Geometry: final body of the model. Coordinates: model frame, mm. A direction names the side the tool comes from. Give positions to 0.01 mm unless a question says otherwise; leave off trailing zeros. Write each loop counter-clockwise with the first axis right and the second up, starting at its lowest first coordinate (ties: lowest second). Pieces come first, ordered by that corner, then holes.
```python
from build123d import *

# Parameters (mm, degrees)
SKETCH1_R                   = 8.89
BOSS_EXTRUDE1_DEPTH         = 33.02
F_1_4_20_TAPPED_HOLE1_D     = 5.1054
F_1_4_20_TAPPED_HOLE1_DEPTH = 12.7
F_1_4_20_TAPPED_HOLE1_TIP   = 1.533816902
F_6_0MM_DOWEL_HOLE1_D       = 6
F_6_0MM_DOWEL_HOLE1_DEPTH   = 17.9999894
F_6_0MM_DOWEL_HOLE1_TIP     = 1.802581857
M4X0_7_TAPPED_HOLE1_REACH   = 40.542
M4X0_7_TAPPED_HOLE1_BORE_R  = 1.65


with BuildPart() as part:
    # Sketch1 → Boss-Extrude1 (new body)
    with BuildSketch(Plane(origin=(0, 0, 0), x_dir=(1, 0, 0), z_dir=(0, 1, 0))):
        with Locations(Location((0, 0, 0), (0, 0, 270))):
            Circle(SKETCH1_R)
    extrude(amount=BOSS_EXTRUDE1_DEPTH)

    # 1/4-20 Tapped Hole1
    with Locations(Plane(origin=(0, 33.02, 0), x_dir=(1, 0, 0), z_dir=(0, 1, 0))):
        with Locations((0, 3.175)):
            Hole(F_1_4_20_TAPPED_HOLE1_D / 2, depth=F_1_4_20_TAPPED_HOLE1_DEPTH)
            with Locations((0, 0, -(F_1_4_20_TAPPED_HOLE1_DEPTH + F_1_4_20_TAPPED_HOLE1_TIP / 2))):  # 118° drill point
                Cone(0, F_1_4_20_TAPPED_HOLE1_D / 2, F_1_4_20_TAPPED_HOLE1_TIP, mode=Mode.SUBTRACT)

    # Ø6.0mm Dowel Hole1
    with Locations(Plane(origin=(0, 0, 0), x_dir=(-1, 0, 0), z_dir=(0, -1, 0))):
        with Locations((0, 0)):
            Hole(F_6_0MM_DOWEL_HOLE1_D / 2, depth=F_6_0MM_DOWEL_HOLE1_DEPTH)
            with Locations((0, 0, -(F_6_0MM_DOWEL_HOLE1_DEPTH + F_6_0MM_DOWEL_HOLE1_TIP / 2))):  # 118° drill point
                Cone(0, F_6_0MM_DOWEL_HOLE1_D / 2, F_6_0MM_DOWEL_HOLE1_TIP, mode=Mode.SUBTRACT)

    # M4x0.7 Tapped Hole1 bore → M4x0.7 Tapped Hole1 (cut, up to next)
    with BuildSketch(Plane(origin=(0, 0, -8.89), x_dir=(-1, 0, 0), z_dir=(0, 0, -1)), mode=Mode.PRIVATE) as m4x0_7_tapped_hole1_sk1:
        with Locations((0, 10)):
            Circle(M4X0_7_TAPPED_HOLE1_BORE_R)
    m4x0_7_tapped_hole1_tool1 = extrude(m4x0_7_tapped_hole1_sk1.sketch, amount=-M4X0_7_TAPPED_HOLE1_REACH, mode=Mode.PRIVATE) & part.part
    add(m4x0_7_tapped_hole1_tool1.solids().sort_by_distance((0, 10, -8.89))[0], mode=Mode.SUBTRACT)


solid = part.part
```
Item 1: Section D-D, the plane y = 30. Return the cut outline in (x, z) (3 decimals).
Found:
outline: circle Ø17.78 at (0, 0); hole circle Ø5.105 at (0, -3.175)
Item 2: Section B-B, the plane y = 7. Return the cut outline in (x, z).
Found:
outline: circle Ø17.78 at (0, 0); hole circle Ø6 at (0, 0)
Item 3: Reachability of faces 1 (the face through (0, 33.02, 0)), 2 (the face through (-1.524, 9.368, -5.743)), 3 (the face through (-1.18, 26.58, -0.91)) from +Z, -Z, +X, -X, +Y, -Y: full face, straight path, thin tool, end or side. Return the list, or none.
Found:
face 1: +Z, -Z, +X, -X, +Y
face 2: -Z
face 3: +Y
Item 4: Pin query (flat end, axial travel): pin 1 Ø1 at (y, z) = (4, 3.5) entering from +X; pin 2 Ø6 at (y, z) = (9.5, 5) entering from -X. Return the tip coordinate at first contact, or that it passes through.
Found:
pin 1: stops at x = 8.37
pin 2: stops at x = -8.66
Item 5: Line query: L1, parallel to Z at x = 0, y = 12.5; L2, parallel to X at y = 9, z = -7; L3, parallel to X at y = 15, z = -2.5. Output: solid intervals per line, ascending.
Found:
L1: z = -8.89 to -3, 3 to 8.89
L2: x = -5.48 to -1.31, 1.31 to 5.48
L3: x = -8.53 to -1.66, 1.66 to 8.53
Item 6: Section A-A, the plane z = -7.5. Return the cut outline in (x, y), plus the area to 3 significant figures.
Found:
outline: (-4.77, 0) - (4.77, 0) - (4.77, 33.02) - (-4.77, 33.02) - close; hole circle Ø3.3 at (0, 10)
area: 307 mm2
Item 7: Section C-C, the plane x = -7.5. Return the cut outline in (y, z).
Found:
outline: (0, -4.77) - (33.02, -4.77) - (33.02, 4.77) - (0, 4.77) - close
Item 8: Pull-direction query (X, two-part tool) for faces 4 (the face through (-4, 0, 0)), 5 (the face through (2.67, 16.28, 8.48)), 6 (the face through (-0.65, 9.13, 2.93)), 7 (the face through (-0.096, 19.053, -2.742)); classes: +X half, -X half, draft (parallel to the pull), parting line (faces both ways), or undercut.
Found:
face 4: draft
face 5: parting line
face 6: undercut
face 7: undercut
